Input: part model. Units: mm. Frame: model coordinates. A direction names the side the tool comes from. Coordinates: 2 decimals unless noted, no trailing zeros. Write each loop counter-clockwise with the first axis right and the second up, starting at its lowest first coordinate (ties: lowest second). Pieces come first, ordered by that corner, then holes. Notation, with made-up numbers: (9, 16.25) - (64, 16.25) arc R24 ccw to (64, 34.25) - close; hole circle Ø10 at (-13, -1.5). An arc over 180 degrees is marked (long way). One line per question, with ' | ' between items. Start each with the question number.
1) Section query C-C on z = 28.5. Return loops of the section in (x, y).
2) Section query A-A on x = 10. Return loops of the section in (y, z), and give its area (3 significant figures).
3) First-contact query: P1, Ø3, axis at x = 11.5, z = 8, coming from the +Y side; P2, Ø4, axis at x = 7.5, z = 13, coming from the -Y side. Flat tips, straight axial feed; report the tip coordinate or a pass-through.
4) Line query: line 1 (Z direction, x = 9.5, y = 8.25); line 2 (X direction, y = 7.5, z = 23); line 3 (X direction, y = 7, z = 27.5). Output: solid intervals per line, ascending.
5) Reachability of faces 1 (the cylindrical face through (11.61, 2.47, 15.79)), 2 (the flat face through (10, 5, 31)) from +Z, -Z, +X, -X, +Y, -Y: full face, straight path, thin tool, end or side. Return the list, or none.
6) Section query B-B on y = 5. Return loops of the section in (x, z), and give its area (3 significant figures).
Autodesk Fusion 360 part; units mm, degrees
sketch "Esboço1" plane through (0, 0, 0) normal (0, 0, 1) x (1, 0, 0)
  circle A0 centre (10, 5) radius 3
  circle A1 centre (10, 5) radius 3.5
  dimension "d1" = 6
  dimension "d2" = 7
extrude "Extrusão1" add sketch "Esboço1" along normal blind 31 contours A0
extrude "Extrusão2" add sketch "Esboço1" along normal blind 1
extrude "Extrusão3" add sketch "Esboço1" against normal blind 1 contours A0 | A1
Answer key:
1) outline: circle Ø6 at (10, 5)
2) outline: (1.5, -1) - (8.5, -1) - (8.5, 1) - (8, 1) - (8, 31) - (2, 31) - (2, 1) - (1.5, 1) - close | area: 194 mm²
3) P1: y = 8 | P2: y = 2.04
4) line 1: -1 to 1 | line 2: 8.34 to 11.66 | line 3: 7.76 to 12.24
5) face 1: +Z | face 2: +Z, +X, -X, +Y, -Y
6) outline: (6.5, -1) - (13.5, -1) - (13.5, 1) - (13, 1) - (13, 31) - (7, 31) - (7, 1) - (6.5, 1) - close | area: 194 mm²
